Part model, mm, in its own coordinate system. A direction names the side the tool comes from. Coordinates: 2 decimals unless noted, no trailing zeros. Order: outer loops, then holes, each group sorted by start corner. A loop starts at its lowest first (then second) coordinate and runs counter-clockwise, first axis right, second up.
1) Cut at D-D (y = 15). List the corners of the cut face in (x, z), and give its area (3 significant figures).
2) Pin check, flat tips, straight feed: pin 1 Ø3 at (x, z) = (1.5, -3) entering from +Y; pin 2 Ø3 at (x, y) = (1, 4) entering from +Z; pin 3 Ø2 at (x, y) = (3.5, 17) entering from -Z; pin 4 Ø3.5 at (y, z) = (5, -7.5) entering from -X. Stop position of each tip, or through.
3) Mould opens along Y. For faces 1 (the flat face through (3, 14, -4)), 2 (the cylindrical face through (2.958, 3.526, -8.852)), 3 (the flat face through (3, 17, -21)), 4 (the cylindrical face through (2.958, 4.566, -25.548)) say: +Y half, -Y half, draft (parallel to the pull), parting line (faces both ways), or undercut.
4) Cut at C-C (z = -27.5). List the corners of the cut face in (x, y), and give its area (3 significant figures).
5) Tool access for faces 5 (the flat face through (3, 17, -14)), 6 (the flat face through (6, 8, -17)), 7 (the flat face through (3, 14, -32)), 8 (the flat face through (3, 17, -7)): list every direction of +Z, -Z, +X, -X, +Y, -Y with a clear straight run to the whole face (end or side of a thin tool).
6) Cut at B-B (x = 2.8). List the corners of the cut face in (y, z), and give its area (3 significant figures).
7) Wall check: L1, parallel to Z at x = 2.1, y = 5; L2, parallel to Z at x = 1.1, y = 15.5; L3, parallel to Z at x = 1.7, y = 6.25. Give the ranges that are in metal, low to high.
8) Cut at A-A (y = 5). List the corners of the cut face in (x, z).
Autodesk Inventor part; units mm, degrees
ref_plane "YZ Plane" through (0, 0, 0) normal (1, 0, 0) x (0, 1, 0)
ref_plane "XZ Plane" through (0, 0, 0) normal (0, 1, 0) x (-1, 0, 0)
ref_plane "XY Plane" through (0, 0, 0) normal (0, 0, 1) x (1, 0, 0)
sketch "Sketch1" plane through (0, 0, 0) normal (1, 0, 0) x (0, 1, 0)
  line L0 (0, 0) -> (20, 0)
  line L1 (20, 0) -> (20, -35)
  line L2 (20, -35) -> (0, -35)
  line L3 (0, -35) -> (0, 0)
  circle A0 centre (5, -7.5) radius 2
  circle A1 centre (5, -27.5) radius 2
  dimension "d0" = 20
  dimension "d1" = 35
  dimension "d5" = 4
  dimension "d6" = 4
extrude "Extrusion1" add sketch "Sketch1" along normal blind 6
sketch "Sketch2" plane through (6, 0, 0) normal (1, 0, 0) x (0, 0, -1)
  line L0 (0, 20) -> (0, 0)
  line L1 (0, 20) -> (7, 20)
  line L2 (7, 20) -> (7, 14)
  line L3 (7, 14) -> (0, 14)
  line L4 (0, 14) -> (0, 20)
  dimension "d9" = 7
  dimension "d10" = 6
extrude "Extrusion2" cut sketch "Sketch2" against normal blind 6
pattern_linear "Rectangular Pattern1" count 3 spacing 14 along (0, 0, -1) of "Extrusion2"
properties part number "g_mount 2"
Geometry check:
1. outline: (0, -28) - (6, -28) - (6, -21) - (0, -21) - close; (0, -14) - (6, -14) - (6, -7) - (0, -7) - close
1. area: 84.0 mm2
2. pin 1: stops at y = 14
2. pin 2: stops at z = 0
2. pin 3: stops at z = -28
2. pin 4: passes through
3. face 1: +Y half
3. face 2: undercut
3. face 3: draft
3. face 4: undercut
4. outline: (0, 0) - (6, 0) - (6, 3) - (0, 3) - close; (0, 7) - (6, 7) - (6, 20) - (0, 20) - close
4. area: 96.0 mm2
5. face 5: +X, -X, +Y
5. face 6: +Z, -Z, +X, +Y, -Y
5. face 7: -Z, +X, -X, +Y
5. face 8: +Z, +X, -X, +Y
6. outline: (0, -35) - (14, -35) - (14, -28) - (20, -28) - (20, -21) - (14, -21) - (14, -14) - (20, -14) - (20, -7) - (14, -7) - (14, 0) - (0, 0) - close; hole circle Ø4 at (5, -27.5); hole circle Ø4 at (5, -7.5)
6. area: 549 mm2
7. L1: z = -35 to -29.5, -25.5 to -9.5, -5.5 to 0
7. L2: z = -28 to -21, -14 to -7
7. L3: z = -35 to -29.06, -25.94 to -9.06, -5.94 to 0
8. outline: (0, -35) - (6, -35) - (6, -29.5) - (0, -29.5) - close; (0, -25.5) - (6, -25.5) - (6, -9.5) - (0, -9.5) - close; (0, -5.5) - (6, -5.5) - (6, 0) - (0, 0) - close
